Could you check a few things on this model? Use its own coordinates, in mm. Face numbers are marked on the shaded views. A direction names the side the tool comes from. Give positions to 0.01 mm unless a question says otherwise; leave off trailing zeros. Loops run counter-clockwise (first coordinate to the right, second up) from the corner with the lowest first, then second, coordinate; pieces in that order, holes last. Notation, with made-up numbers: (0, -0.75) -> (54, -0.75) arc R11 cw to (54, 8.25) -> close; hole circle Ø6 at (65.5, 61). An arc over 180 degrees is marked (long way). Write each question's results on one line, items separated by ' | '. Start each with the question number.
Q1. We'd pull the mould along Y, two halves only. Please class the marked faces 3, 4, 5 and 6: released by +Y, released by -Y, zero draft, split by the parting line, or undercut.
Q2. If we section it at B-B, the plane y = 0: List the corners of the cut face in (x, z) for me.
Q3. If we section it at A-A, the plane x = 0: List the corners of the cut face in (y, z) for me.
Q4. If we section it at C-C, the plane z = 42.5: List the corners of the cut face in (x, y) for me.
Q5. Which directions (+Z, -Z, +X, -X, +Y, -Y) give clear straight access to the entire face, cutting with the end or side of a thin tool? Please do the marked faces 1 and 2.
Q6. If we section it at D-D, the plane z = 16: List the corners of the cut face in (x, y) for me (3 decimals).
Q7. Will these pins go through, and if not, where does the flat tip stop? P1, Ø8, axis at x = -10, y = -23, coming from the -Z side; P2, Ø5.5, axis at x = 0, y = -41.75, coming from the +Z side; P3, Ø1.5, axis at x = 35.5, z = 23.5, coming from the -Y side; P4, Ø20, axis at x = 0, y = 0, coming from the -Z side.
Q8. If I drill on line 1 along Y through (x, z) = (0, 15.25); line 2 along Y through (x, z) = (2, 11.5); line 3 along Y through (x, z) = (0, 41), over which ranges is the centre line in solid material (lowest first)?
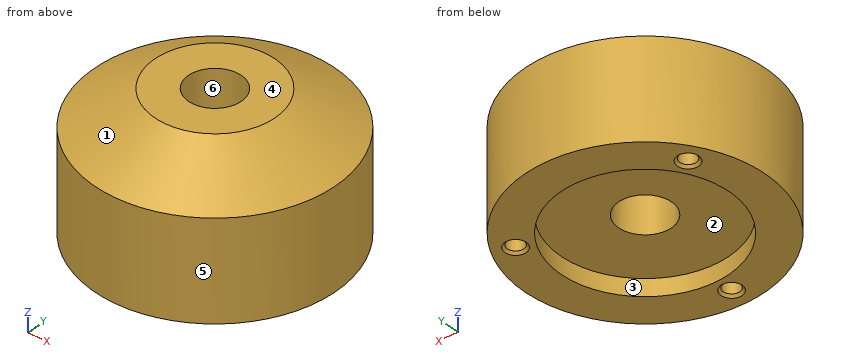
from build123d import *

# Parameters (mm, degrees)
SKETCH_R        = 50
PAD_DEPTH       = 56
SKETCH004_R     = 11
POCKET_DEPTH    = 56.001
SKETCH003_R     = 35
POCKET001_DEPTH = 7
CHAMFER_SIZE2   = 25
CHAMFER_SIZE    = 15
SKETCH005_R     = 3.4
POCKET002_DEPTH = 20
CHAMFER001_SIZE = 1


with BuildPart() as part:
    # Sketch → Pad (new body)
    with BuildSketch(Plane.XY):
        Circle(SKETCH_R)
    extrude(amount=PAD_DEPTH)

    # Sketch004 → Pocket (cut, through all)
    with BuildSketch(Plane.XY):
        Circle(SKETCH004_R)
    extrude(amount=POCKET_DEPTH, mode=Mode.SUBTRACT)

    # Sketch003 → Pocket001 (cut)
    with BuildSketch(Plane(origin=(0, 0, 0), x_dir=(1, 0, 0), z_dir=(0, 0, -1))):
        Circle(SKETCH003_R)
    extrude(amount=-POCKET001_DEPTH, mode=Mode.SUBTRACT)

    # Chamfer
    chamfer_edges = [part.edges().sort_by_distance(p)[0] for p in [
        (-50, 0, 56),
    ]]
    chamfer_side = part.faces().sort_by_distance((-50, 0, 28))[0]
    chamfer(chamfer_edges, length=CHAMFER_SIZE, length2=CHAMFER_SIZE2, reference=chamfer_side)

    # Sketch005 (on Face3 of Chamfer) → Pocket002 (cut)
    with BuildSketch(Plane(origin=(0, 0, 0), x_dir=(1, 0, 0), z_dir=(0, 0, -1))):
        with Locations((0, 41.75)):
            Circle(SKETCH005_R)
        with Locations((36.156561, -20.875)):
            Circle(SKETCH005_R)
        with Locations((-36.156561, -20.875)):
            Circle(SKETCH005_R)
    extrude(amount=-POCKET002_DEPTH, mode=Mode.SUBTRACT)

    # Chamfer001
    chamfer001_edges = [part.edges().sort_by_distance(p)[0] for p in [
        (32.756561, 20.875, 0),
        (-3.4, -41.75, 0),
        (-39.556561, 20.875, 0),
    ]]
    chamfer(chamfer001_edges, length=CHAMFER001_SIZE)


solid = part.part
Final values:
1) face 3: undercut | face 4: zero draft | face 5: split by the parting line | face 6: undercut
2) outline: (-50, 0) -> (-35, 0) -> (-35, 7) -> (-11, 7) -> (-11, 56) -> (-25, 56) -> (-50, 41) -> close; (11, 7) -> (35, 7) -> (35, 0) -> (50, 0) -> (50, 41) -> (25, 56) -> (11, 56) -> close
3) outline: (-50, 0) -> (-46.15, 0) -> (-45.15, 1) -> (-45.15, 20) -> (-38.35, 20) -> (-38.35, 1) -> (-37.35, 0) -> (-35, 0) -> (-35, 7) -> (-11, 7) -> (-11, 56) -> (-25, 56) -> (-50, 41) -> close; (11, 7) -> (35, 7) -> (35, 0) -> (50, 0) -> (50, 41) -> (25, 56) -> (11, 56) -> close
4) outline: circle Ø95 at (0, 0); hole circle Ø22 at (0, 0)
5) face 1: +Z | face 2: -Z
6) outline: circle Ø100 at (0, 0); hole circle Ø6.8 at (-36.157, 20.875); hole circle Ø22 at (0, 0); hole circle Ø6.8 at (0, -41.75); hole circle Ø6.8 at (36.157, 20.875)
7) P1: stops at z = 7 | P2: stops at z = 47.6 | P3: stops at y = -35.95 | P4: passes through
8) line 1: y = -50 to -45.15, -38.35 to -11, 11 to 50 | line 2: y = -49.96 to -44.5, -39 to -10.82, 10.82 to 49.96 | line 3: y = -50 to -11, 11 to 50
